CAD build for the part. Positions are in the model's coordinates, mm. Give positions to 0.01 mm unless a question says otherwise; leave off trailing zeros. Order: outer loops, then holes, each group sorted by start corner. A loop starts at its lowest first (then second) coordinate and runs counter-clockwise, first axis right, second up. Notation, with made-up numbers: (30.25, 35) -> (49.25, 35) arc R30 cw to (49.25, 59) -> close; hole circle Ø8 at (57, 83). An arc over 180 degrees is marked (long way). Answer as CSV lines item,"result".
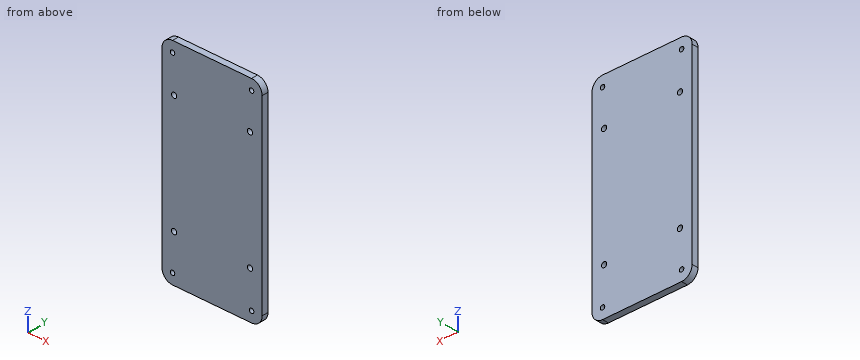
```python
from build123d import *

# Parameters (mm, degrees)
SKETCH1_R           = 2.5
SKETCH1_R_2         = 2.125
BOSS_EXTRUDE1_DEPTH = 6.096


with BuildPart() as part:
    # Sketch1 → Boss-Extrude1 (new body)
    with BuildSketch(Plane(origin=(0, 0, 0), x_dir=(1, 0, 0), z_dir=(0, 1, 0))):
        with BuildLine():
            Line((-37.5, 100.5), (37.5, 100.5))
            ThreePointArc((37.5, 100.5), (44.571067812, 97.571067812), (47.5, 90.5))
            Line((47.5, 90.5), (47.5, -90.5))
            ThreePointArc((47.5, -90.5), (44.571067812, -97.571067812), (37.5, -100.5))
            Line((37.5, -100.5), (-37.5, -100.5))
            ThreePointArc((-37.5, -100.5), (-44.571067812, -97.571067812), (-47.5, -90.5))
            Line((-47.5, -90.5), (-47.5, 90.5))
            ThreePointArc((-47.5, 90.5), (-44.571067812, 97.571067812), (-37.5, 100.5))
        make_face()
        with Locations(Location((-36, 56, 0), (0, 0, 90))):
            Circle(SKETCH1_R, mode=Mode.SUBTRACT)
        with Locations(Location((36, 56, 0), (0, 0, 90))):
            Circle(SKETCH1_R, mode=Mode.SUBTRACT)
        with Locations(Location((36, -56, 0), (0, 0, 90))):
            Circle(SKETCH1_R, mode=Mode.SUBTRACT)
        with Locations(Location((-36, -56, 0), (0, 0, 90))):
            Circle(SKETCH1_R, mode=Mode.SUBTRACT)
        with Locations(Location((-37.5, 90.5, 0), (0, 0, 90))):
            Circle(SKETCH1_R_2, mode=Mode.SUBTRACT)
        with Locations(Location((37.5, 90.5, 0), (0, 0, 90))):
            Circle(SKETCH1_R_2, mode=Mode.SUBTRACT)
        with Locations(Location((37.5, -90.5, 0), (0, 0, 90))):
            Circle(SKETCH1_R_2, mode=Mode.SUBTRACT)
        with Locations(Location((-37.5, -90.5, 0), (0, 0, 90))):
            Circle(SKETCH1_R_2, mode=Mode.SUBTRACT)
    extrude(amount=BOSS_EXTRUDE1_DEPTH)


solid = part.part
```
1) Band-saw the part on A-A, the plane z = -56. Write the cut outline in (x, y).
Data:
outline,"(-47.5, 0) -> (-38.5, 0) -> (-38.5, 6.1) -> (-47.5, 6.1) -> close; (-33.5, 0) -> (33.5, 0) -> (33.5, 6.1) -> (-33.5, 6.1) -> close; (38.5, 0) -> (47.5, 0) -> (47.5, 6.1) -> (38.5, 6.1) -> close"
2) Pin check, flat tips, straight feed: P1, Ø8, axis at x = 10.5, z = 44, coming from the -Y side; P2, Ø4.5, axis at x = 36, z = -56, coming from the +Y side. Stop position of each tip, or through.
Data:
P1,"stops at y = 0"
P2,"passes through"
3) Wall check: line 1 along X through (y, z) = (2, -90.5) (3 decimals); line 2 along X through (y, z) = (2.75, 56); line 3 along Z through (x, y) = (37.5, 3) (3 decimals). Give the ranges that are in metal, low to high. Write a range as [from, to].
Data:
line 1,"x = [-47.5, -39.625], [-35.375, 35.375], [39.625, 47.5]"
line 2,"x = [-47.5, -38.5], [-33.5, 33.5], [38.5, 47.5]"
line 3,"z = [-100.5, -92.625], [-88.375, -58], [-54, 54], [58, 88.375], [92.625, 100.5]"
